Could you check a few things on this drawing? It's one solid part, dimensions in mm from its lowest x, y, z. Give positions to 0.01 mm unless a question says otherwise; leave off trailing zeros. Loops run counter-clockwise (first coordinate to the right, second up) from the corner with the lowest first, then second, coordinate; pieces in that order, holes last. Notation, with made-up numbers: (-11, -6.75) - (25, -6.75) arc R12 ccw to (25, 0.25) - close; hole circle Ø2 at (64.25, 64). An arc over 180 degrees is marked (long way). Write item = value, one per line.
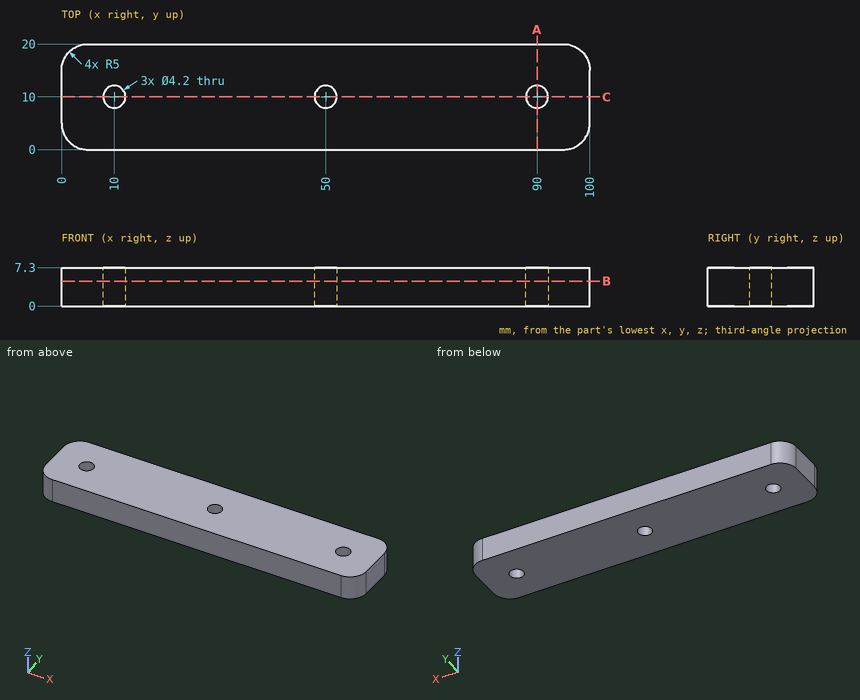
Q1. Imagine slicing it at A-A, the plane x = 90. Write out the boundary of the cut face in (y, z).
Output:
outline = (0, 0) - (7.9, 0) - (7.9, 7.3) - (0, 7.3) - close; (12.1, 0) - (20, 0) - (20, 7.3) - (12.1, 7.3) - close
Q2. Imagine slicing it at B-B, the plane z = 4.75. Write out the boundary of the cut face in (x, y).
Output:
outline = (0, 5) arc R5 ccw to (5, 0) - (95, 0) arc R5 ccw to (100, 5) - (100, 15) arc R5 ccw to (95, 20) - (5, 20) arc R5 ccw to (0, 15) - close; hole circle Ø4.2 at (10, 10); hole circle Ø4.2 at (50, 10); hole circle Ø4.2 at (90, 10)
Q3. I need wall thicknesses on L1, parallel to Y at x = 10, z = 4.25; L2, parallel to X at y = 11.5, z = 6.25; L3, parallel to Y at x = 48.5, z = 1.75. Which ranges of each line are inside material? Lowest first, please.
Output:
L1 = 0 to 7.9, 12.1 to 20
L2 = 0 to 8.53, 11.47 to 48.53, 51.47 to 88.53, 91.47 to 100
L3 = 0 to 8.53, 11.47 to 20
Q4. Imagine slicing it at C-C, the plane y = 10. Write out the boundary of the cut face in (x, z), then the cut area to 3 significant figures.
Output:
outline = (0, 0) - (7.9, 0) - (7.9, 7.3) - (0, 7.3) - close; (12.1, 0) - (47.9, 0) - (47.9, 7.3) - (12.1, 7.3) - close; (52.1, 0) - (87.9, 0) - (87.9, 7.3) - (52.1, 7.3) - close; (92.1, 0) - (100, 0) - (100, 7.3) - (92.1, 7.3) - close
area = 638 mm2
Q5. For pin 1 (6.5 mm diameter, centred on x = 50, y = 10, fed in from +Z), with a flat end and sliding along its axis, tell me the tip position at first contact or that it passes through.
Output:
pin_1 = 7.3
